Verification items for this drawing (mm, ordinates from the low corner). A direction names the side the tool comes from. Round coordinates to 2 decimals unless told otherwise and drop trailing zeros. Order: outer loops, then holes, each group sorted by start corner. A loop starts at its lowest first (then second) coordinate and runs counter-clockwise, first axis right, second up. Notation, with made-up numbers: M -19,59.5 L 4,59.5 A21 ccw 4,79.5 Z; hole C 1,58 d4. An arc over 180 degrees is marked long. One line per item, written item: value. Start each with the question number.
(1) Cross-section at B-B, the plane y = 3.5. Enter the section's corners in (x, z).
(2) Cross-section at C-C, the plane z = 0.75. Enter the section's corners in (x, y), and give its area (3 significant figures).
(3) Thickness scan on L1, parallel to Y at x = 26.5, z = 0.75; L2, parallel to Z at x = 9.5, y = 2.5; L3, parallel to Y at x = 19, z = 4.5. Record the ranges inside material, lowest first.
(4) Depth check by flat-ended pin: pin 1 Ø1.5 at (x, y) = (7, 4.5) entering from -Z; pin 2 Ø4 at (x, z) = (22.5, 2) entering from -Y. Enter the tip coordinate at first touch or a pass-through.
(5) Cross-section at A-A, the plane x = 8. Enter the section's corners in (y, z), and give its area (3 significant figures).
(6) Access from +Z, -Z, +X, -X, +Y, -Y to the whole of each face (thin tool, end or side, straight path). Record for the marked faces 1 and 2.
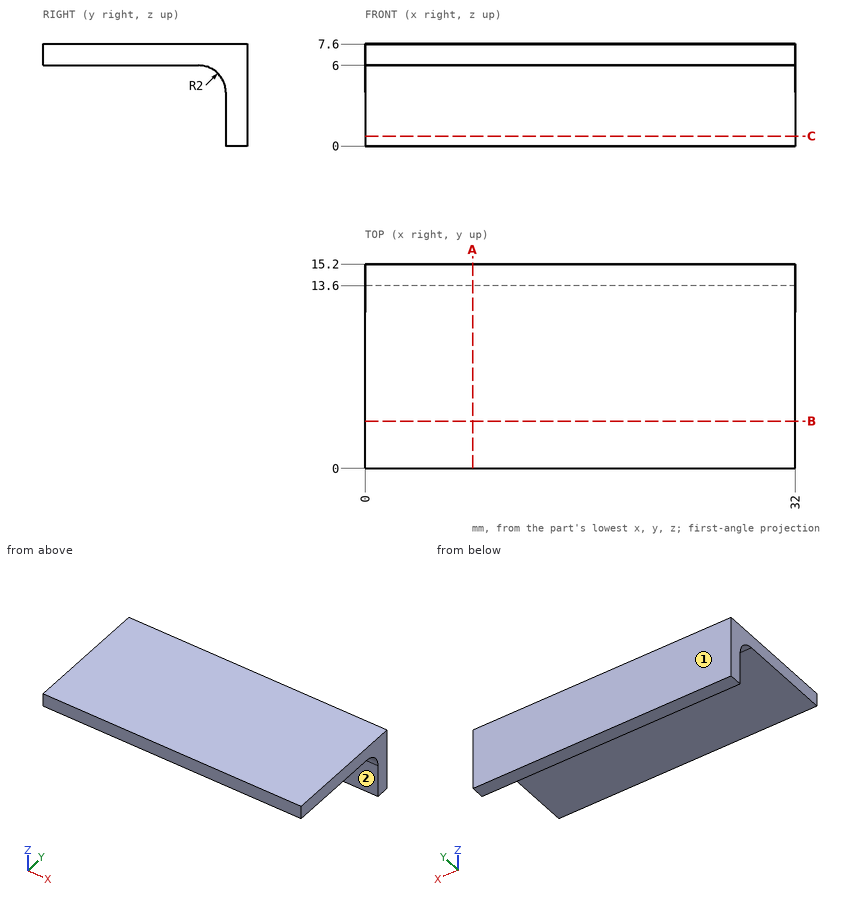
Values found:
1. outline: M 0,6 L 32,6 L 32,7.6 L 0,7.6 Z
2. outline: M 0,13.6 L 32,13.6 L 32,15.2 L 0,15.2 Z
2. area: 51.2 mm^2
3. L1: 13.6 to 15.2
3. L2: 6 to 7.6
3. L3: 13.54 to 15.2
4. pin 1: z = 6
4. pin 2: y = 13.6
5. outline: M 0,6 L 11.6,6 A2 cw 13.6,4 L 13.6,0 L 15.2,0 L 15.2,7.6 L 0,7.6 Z
5. area: 34.8 mm^2
6. face 1: +Z, -Z, +X, -X, +Y
6. face 2: -Z, +X, -X, -Y
